Here's how the part is built. I have some questions about the finished solid (model axes, mm). A direction names the side the tool comes from. Coordinates: 2 decimals unless noted, no trailing zeros. Loops run counter-clockwise (first coordinate to the right, second up) from the corner with the lowest first, then second, coordinate; pieces in that order, holes last. Notation, with made-up numbers: (29, 17) - (61, 17) arc R17 ccw to (61, 25) - close; hole circle Ø7 at (-12.75, -32.5). An arc over 180 degrees is marked (long way). Use a Markdown table: item, result.
```python
from build123d import *

# Parameters (mm, degrees)
SKETCH1_W           = 125
SKETCH1_H           = 245
BOSS_EXTRUDE1_DEPTH = 5
SKETCH2_W           = 15
SKETCH2_H           = 30
BOSS_EXTRUDE2_DEPTH = 5
SKETCH3_R           = 2.5
CUT_EXTRUDE1_DEPTH  = 158.368235883
SKETCH4_R           = 1.75
CUT_EXTRUDE2_DEPTH  = 158.368235883
FILLET4_R           = 7.5


with BuildPart() as part:
    # Sketch1 → Boss-Extrude1 (new body)
    with BuildSketch(Plane(origin=(0, 0, 0), x_dir=(1, 0, 0), z_dir=(0, 1, 0))):
        with Locations((-8.498498498, 9.196696697)):
            Rectangle(SKETCH1_W, SKETCH1_H)
    extrude(amount=BOSS_EXTRUDE1_DEPTH)

    # Sketch2 → Boss-Extrude2 (add)
    with BuildSketch(Plane(origin=(0, 5, 0), x_dir=(1, 0, 0), z_dir=(0, 1, 0))):
        with Locations((61.501501502, 116.696696697)):
            Rectangle(SKETCH2_W, SKETCH2_H)
        with Locations((-78.498498498, 116.696696697)):
            Rectangle(SKETCH2_W, SKETCH2_H)
        with Locations((-78.498498498, -98.303303303)):
            Rectangle(SKETCH2_W, SKETCH2_H)
        with Locations((61.501501502, -98.303303303)):
            Rectangle(SKETCH2_W, SKETCH2_H)
    extrude(amount=-BOSS_EXTRUDE2_DEPTH)

    # Sketch3 → Cut-Extrude1 (cut, through all)
    with BuildSketch(Plane.XZ):
        with Locations(Location((-78.498498498, 98.303303303, 0), (0, 0, 270))):
            Circle(SKETCH3_R)
        with Locations(Location((61.501501502, 98.303303303, 0), (0, 0, 270))):
            Circle(SKETCH3_R)
        with Locations(Location((-78.498498498, -116.696696697, 0), (0, 0, 270))):
            Circle(SKETCH3_R)
        with Locations(Location((61.501501502, -116.696696697, 0), (0, 0, 270))):
            Circle(SKETCH3_R)
    extrude(amount=-CUT_EXTRUDE1_DEPTH, mode=Mode.SUBTRACT)

    # Sketch4 → Cut-Extrude2 (cut, through all)
    with BuildSketch(Plane(origin=(0, 5, 0), x_dir=(1, 0, 0), z_dir=(0, 1, 0))):
        with Locations(Location((46.501501502, 124.196696697, 0), (0, 0, 270))):
            Circle(SKETCH4_R)
        with BuildLine():
            Line((44.751501502, -83.553303303), (44.751501502, -78.553303303))
            ThreePointArc((44.751501502, -78.553303303), (46.501501502, -76.803303303), (48.251501502, -78.553303303))
            Line((48.251501502, -78.553303303), (48.251501502, -83.553303303))
            ThreePointArc((48.251501502, -83.553303303), (46.501501502, -85.303303303), (44.751501502, -83.553303303))
        make_face()
        with BuildLine():
            Line((-65.248498498, -108.553303303), (-65.248498498, -103.553303303))
            ThreePointArc((-65.248498498, -103.553303303), (-63.498498498, -101.803303303), (-61.748498498, -103.553303303))
            Line((-61.748498498, -103.553303303), (-61.748498498, -108.553303303))
            ThreePointArc((-61.748498498, -108.553303303), (-63.498498498, -110.303303303), (-65.248498498, -108.553303303))
        make_face()
        with BuildLine():
            Line((-65.248498498, 27.446696697), (-65.248498498, 32.446696697))
            ThreePointArc((-65.248498498, 32.446696697), (-63.498498498, 34.196696697), (-61.748498498, 32.446696697))
            Line((-61.748498498, 32.446696697), (-61.748498498, 27.446696697))
            ThreePointArc((-61.748498498, 27.446696697), (-63.498498498, 25.696696697), (-65.248498498, 27.446696697))
        make_face()
        with BuildLine():
            Line((-65.248498498, 102.446696697), (-65.248498498, 107.446696697))
            ThreePointArc((-65.248498498, 107.446696697), (-63.498498498, 109.196696697), (-61.748498498, 107.446696697))
            Line((-61.748498498, 107.446696697), (-61.748498498, 102.446696697))
            ThreePointArc((-61.748498498, 102.446696697), (-63.498498498, 100.696696697), (-65.248498498, 102.446696697))
        make_face()
    extrude(amount=-CUT_EXTRUDE2_DEPTH, mode=Mode.SUBTRACT)

    # Fillet4
    fillet4_edges = [part.edges().sort_by_distance(p)[0] for p in [
        (-70.998498498, 2.5, 83.303303303),
        (-85.998498498, 2.5, 83.303303303),
        (-85.998498498, 2.5, 113.303303303),
        (69.001501502, 2.5, 113.303303303),
        (69.001501502, 2.5, 83.303303303),
        (54.001501502, 2.5, 83.303303303),
        (54.001501502, 2.5, -101.696696697),
        (69.001501502, 2.5, -101.696696697),
        (69.001501502, 2.5, -131.696696697),
        (-85.998498498, 2.5, -131.696696697),
        (-70.998498498, 2.5, -101.696696697),
        (-85.998498498, 2.5, -101.696696697),
    ]]
    fillet(fillet4_edges, radius=FILLET4_R - 0.0001)  # a hair under: the kernel refuses the full size


solid = part.part
```
Q1. Please list where these lines run through material, in increasing order: L1, parallel to Z at x = 60.5, y = 2.4; L2, parallel to X at y = 3.35, z = 99.5; L3, parallel to X at y = 1.8, z = 100. Write a range as from..to.
Check values:
| item | result |
|---|---|
| L1 | -131.7..-118.99, -114.41..-101.63, 83.24..96.01, 100.59..113.3 |
| L2 | -86..-80.69, -76.3..59.31, 63.7..69 |
| L3 | -86..-80.33, -76.66..59.67, 63.34..69 |
Q2. I want a section at B-B, the plane y = 2.95. Give the number of separate pieces and of enclosed holes in the cut face, then the cut area to 3 significant figures.
Check values:
| item | result |
|---|---|
| separate pieces | 1 |
| enclosed holes | 9 |
| area | 32,200 mm^2 |
Q3. I want a section at A-A, the plane z = 9.5. Write out the boundary of the cut face in (x, y).
Check values:
| item | result |
|---|---|
| outline | (-71, 0) - (54, 0) - (54, 5) - (-71, 5) - close |
Q4. If we mould it in two halves opening along Z, with no side actions, what happens to faces 1 (the face through (56.3, 2.5, -99.6)), 2 (the face through (-9, 2, 113.303)), 3 (the face through (69.002, 3, 98))? For each: pulls with the +Z half, pulls with the -Z half, needs draft (parallel to the pull), parting line crosses it, or undercut.
Check values:
| item | result |
|---|---|
| face 1 | undercut |
| face 2 | pulls with the +Z half |
| face 3 | needs draft |
Q5. Which directions (+Z, -Z, +X, -X, +Y, -Y) give clear straight access to the entire face, cutting with the end or side of a thin tool? Please do faces 4 (the face through (66.863, 2.465, -129.441)), 5 (the face through (-83.7, 2.5, -129.6)), 6 (the face through (66.746, 2.465, 85.442)), 7 (the face through (-65.248, 3, -30)), 8 (the face through (-73.14, 2.46, 81.05)).
Check values:
| item | result |
|---|---|
| face 4 | -Z, +X, +Y, -Y |
| face 5 | -Z, -X, +Y, -Y |
| face 6 | +X, +Y, -Y |
| face 7 | +Y, -Y |
| face 8 | -X, +Y, -Y |
Q6. Will these pins go through, and if not, where does the flat tip stop? P1, Ø4, axis at x = -78.5, z = 98.3, coming from the +Y side; P2, Ø1.5, axis at y = 3.5, z = 80, coming from the +X side; P3, Ø2.5, axis at y = 1.5, z = 81.5, coming from the -X side; P4, Ø8, axis at x = 43, z = -42, coming from the -Y side.
Check values:
| item | result |
|---|---|
| P1 | through |
| P2 | x = 55.86 |
| P3 | x = -75.67 |
| P4 | y = 0 |
